For this review, take the finished solid that the model builds, in its own axes (mm). Face numbers are marked on the shaded views. A direction names the side the tool comes from. Round coordinates to 2 decimals unless told otherwise and drop trailing zeros. Loops run counter-clockwise (first coordinate to the right, second up) from the corner with the lowest first, then second, coordinate; pieces in that order, holes last.
1. Clearance check with flat-ended pins moving along their axes: pin 1 Ø1 at (x, z) = (-1.5, -6) entering from -Y; pin 2 Ø1 at (y, z) = (-1.5, -1.5) entering from -X. State where each tip first meets the part, or that it passes through.
2. Consider section C-C on z = -5.5. State the section outline as (x, y) points.
3. To check wall thickness, follow line 1 along Z through (x, y) = (-0.9, -1.65); line 2 along X through (y, z) = (-0.95, -6.75); line 3 along Z through (x, y) = (2.4, -0.5). State the ranges of each line that lie inside material, in increasing order.
4. Tool access review of the marked faces 1 and 2: name each direction out of +Z, -Z, +X, -X, +Y, -Y from which nothing blocks a thin tool from reaching the whole face with its end or side.
5. Consider section D-D on z = 0.75. State the section outline as (x, y) points.
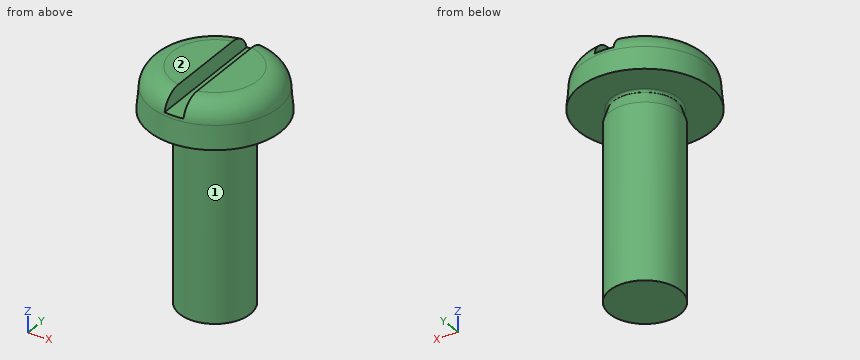
Solid Edge part; units mm, degrees
sketch "Sketch1" plane through (0, 0, 0) normal (0, -1, 0) x (1, 0, 0)
  line L0 (0, -8) -> (1.5, -8)
  line L1 (1.5, -8) -> (1.5, -0.601)
  line L2 (1.5, -0.601) -> (1.3375, -0.101)
  line L3 (1.3375, -0.101) -> (1.3375, 0)
  line L4 (1.3375, 0) -> (2.8, 0)
  line L5 (2.8, 0) -> (2.6425, 1.8)
  line L6 (2.6425, 1.8) -> (0, 1.8)
  dimension "D1" = 1.3375
  dimension "D2" = 1.5
  dimension "D3" = 2.6425
revolve "RevolvedProtrusion1" add sketch "Sketch1" angle 360 about axis through (0, 0, 6) along (0, 0, -1)
fillet "Round_1" radius 0.9 1 edges at (-2.6425, 0, 1.8)
sketch "Sketch2" plane through (0, 0, 0) normal (0, -1, 0) x (1, 0, 0)
  line L0 (-0.4, 1.8) -> (-0.4, 1.1)
  line L1 (-0.4, 1.1) -> (0.4, 1.1)
  line L2 (0.4, 1.1) -> (0.4, 1.8)
  line L3 (0.4, 1.8) -> (-0.4, 1.8)
  dimension "D1" = 0.4
  dimension "D2" = 0.4
extrude "ExtrudedCutout_1" cut sketch "Sketch2" along normal mid plane 5.6
cosmetic_thread "Thread_1" thread depth 7.399
fillet "Round_2" radius 0.1 1 edges at (-1.3375, 0, 0)
chamfer "Chamfer_1" distance 0.0012 angle 30 1 edges at (-1.5, 0, -8) measured on face at (1.03, 0.97, -8)
properties material "Steel"
Resolved:
1. pin 1: stops at y = -1.12
1. pin 2: stops at x = -1.12
2. outline: circle Ø3 at (0, 0)
3. line 1: z = 0 to 1.8
3. line 2: x = -1.16 to 1.16
3. line 3: z = 0 to 1.54
4. face 1: -Z
4. face 2: +Z, +X, -X, +Y, -Y
5. outline: circle Ø5.47 at (0, 0)
